from build123d import *

# Parameters (mm, degrees)
SKETCH1_W                 = 610
SKETCH1_H                 = 410
SKETCH1_W_2               = 580
SKETCH1_H_2               = 380
BOSS_EXTRUDE1_DEPTH       = 25
BOSS_EXTRUDE2_DEPTH       = 15
BOSS_EXTRUDE6_DEPTH       = 15
BOSS_EXTRUDE11_DEPTH      = 25
SKETCH8_W                 = 15
SKETCH8_H                 = 130
BOSS_EXTRUDE12_DEPTH      = 25
SKETCH9_W                 = 15
SKETCH9_H                 = 130
BOSS_EXTRUDE13_DEPTH      = 25
SKETCH10_W                = 150
SKETCH10_H                = 25
BOSS_EXTRUDE14_DEPTH      = 15
SKETCH13_W                = 215
SKETCH13_H                = 25
BOSS_EXTRUDE15_DEPTH      = 15
SKETCH14_W                = 215
SKETCH14_H                = 25
BOSS_EXTRUDE16_DEPTH      = 15
BOSS_EXTRUDE17_DEPTH      = 25
BOSS_EXTRUDE17_DEPTH_BACK = 25
BOSS_EXTRUDE17_START      = -205
SKETCH17_W                = 15
SKETCH17_H                = 150
BOSS_EXTRUDE18_DEPTH      = 25
LOFT13_START              = -525.0000001
LOFT13_DEPTH              = 225.0000002
LOFT13_START_2            = -152.5000001
LOFT13_2_DEPTH            = 415.5000001


with BuildPart() as part:
    # Sketch1 → Boss-Extrude1 (new body)
    with BuildSketch(Plane(origin=(0, 0, 0), x_dir=(1, 0, 0), z_dir=(0, 1, 0))):
        with Locations((695.4, -52.5)):
            Rectangle(SKETCH1_W, SKETCH1_H)
        with Locations((695.4, -52.5)):
            Rectangle(SKETCH1_W_2, SKETCH1_H_2, mode=Mode.SUBTRACT)
    extrude(amount=-BOSS_EXTRUDE1_DEPTH)

    # Sketch2 → Boss-Extrude2 (add)
    with BuildSketch(Plane.XY.offset(257.5)):
        Polygon((1000.4, 0), (1000.4, -290), (1190.4, -290), (1190.4, -500), (1165.4, -500), (1165.4, -315), (1000.4, -315), (1000.4, -500), (975.4, -500), (975.4, 0), align=None)
    extrude(amount=-BOSS_EXTRUDE2_DEPTH)

    # Sketch4 → Boss-Extrude6 (add)
    with BuildSketch(Plane(origin=(0, 0, -152.5), x_dir=(-1, 0, 0), z_dir=(0, 0, -1))):
        Polygon((-1000.4, -500), (-1000.4, -315), (-1165.4, -315), (-1165.4, -500), (-1190.4, -500), (-1190.4, -290), (-1000.4, -290), (-1000.4, 0), (-975.4, 0), (-975.4, -500), align=None)
    extrude(amount=-BOSS_EXTRUDE6_DEPTH)

    # Sketch6 → Boss-Extrude11 (add)
    with BuildSketch(Plane(origin=(0, -290, 0), x_dir=(1, 0, 0), z_dir=(0, 1, 0))):
        Polygon((1700.4, 22.5), (1715.4, 22.5), (1715.4, -52.5), (1715.4, -127.5), (1700.4, -127.5), (1190.4, -257.5), (1190.4, -242.5), (1700.4, -112.5), (1700.4, 7.5), (1190.4, 137.5), (1190.4, 152.5), align=None)
    extrude(amount=-BOSS_EXTRUDE11_DEPTH)

    # Sketch8 → Boss-Extrude12 (add)
    with BuildSketch(Plane.XY.offset(127.5)):
        with Locations((1707.9, -355)):
            Rectangle(SKETCH8_W, SKETCH8_H)
    extrude(amount=-BOSS_EXTRUDE12_DEPTH)

    # Sketch9 → Boss-Extrude13 (add)
    with BuildSketch(Plane(origin=(0, 0, -22.5), x_dir=(-1, 0, 0), z_dir=(0, 0, -1))):
        with Locations((-1707.9, -355)):
            Rectangle(SKETCH9_W, SKETCH9_H)
    extrude(amount=-BOSS_EXTRUDE13_DEPTH)

    # Sketch10 → Boss-Extrude14 (add)
    with BuildSketch(Plane.ZY.offset(-1700.4)):
        with Locations((52.5, -407.5)):
            Rectangle(SKETCH10_W, SKETCH10_H)
    extrude(amount=-BOSS_EXTRUDE14_DEPTH)

    # Sketch13 → Boss-Extrude15 (add)
    with BuildSketch(Plane(origin=(0, 0, -152.5), x_dir=(-1, 0, 0), z_dir=(0, 0, -1))):
        with Locations((-1082.9, -512.5)):
            Rectangle(SKETCH13_W, SKETCH13_H)
    extrude(amount=-BOSS_EXTRUDE15_DEPTH)

    # Sketch14 → Boss-Extrude16 (add)
    with BuildSketch(Plane.XY.offset(257.5)):
        with Locations((1082.9, -512.5)):
            Rectangle(SKETCH14_W, SKETCH14_H)
    extrude(amount=-BOSS_EXTRUDE16_DEPTH)

    # Sketch12 → Loft2 section 0
    with BuildSketch(Plane(origin=(1715.4, 0, 0), x_dir=(0, 0, -1), z_dir=(1, 0, 0))):
        with BuildLine():
            Line((22.5, -420), (22.5, -395))
            Line((22.5, -395), (7.5, -395))
            Line((7.5, -395), (7.5, -420))
            Line((7.5, -420), (22.5, -420))
        make_face()
    # Sketch15 → Loft2 section 1
    with BuildSketch(Plane(origin=(1190.4, 0, 0), x_dir=(0, 0, -1), z_dir=(1, 0, 0))):
        with BuildLine():
            Line((152.5, -525), (137.5, -525))
            Line((137.5, -525), (137.5, -500))
            Line((137.5, -500), (152.5, -500))
            Line((152.5, -500), (152.5, -525))
        make_face()
    loft()

    # Sketch18 → Loft3 section 0
    with BuildSketch(Plane(origin=(1715.4, 0, 0), x_dir=(0, 0, -1), z_dir=(1, 0, 0))):
        with BuildLine():
            Line((-127.5, -420), (-112.5, -420))
            Line((-112.5, -420), (-112.5, -395))
            Line((-112.5, -395), (-127.5, -395))
            Line((-127.5, -395), (-127.5, -420))
        make_face()
    # Sketch19 → Loft3 section 1
    with BuildSketch(Plane(origin=(1190.4, 0, 0), x_dir=(0, 0, -1), z_dir=(1, 0, 0))):
        with BuildLine():
            Line((-257.5, -525), (-242.5, -525))
            Line((-242.5, -525), (-242.5, -500))
            Line((-242.5, -500), (-257.5, -500))
            Line((-257.5, -500), (-257.5, -525))
        make_face()
    loft()



with BuildPart() as body_2:
    # Sketch17 → Boss-Extrude17 (new, two sides: drawn at the far end of the back side and taken through both)
    with BuildSketch(Plane.XY.offset(257.5).offset(BOSS_EXTRUDE17_START - BOSS_EXTRUDE17_DEPTH_BACK)):
        with Locations((-912.1, -250)):
            Rectangle(SKETCH17_W, SKETCH17_H)
    extrude(amount=BOSS_EXTRUDE17_DEPTH + BOSS_EXTRUDE17_DEPTH_BACK)


with BuildPart() as part_1:
    add(part.part)

    add(body_2.part)  # Loft6 merges body 2
    # Sketch21 → Loft6 section 0
    with BuildSketch(Plane(origin=(-904.6, 0, 0), x_dir=(0, 0, -1), z_dir=(1, 0, 0))):
        with BuildLine():
            Line((-77.5, -175), (-62.5, -175))
            Line((-62.5, -175), (-62.5, -200))
            Line((-62.5, -200), (-77.5, -200))
            Line((-77.5, -200), (-77.5, -175))
        make_face()
    # Sketch20 → Loft6 section 1
    with BuildSketch(Plane.ZY.offset(-390.4)):
        with BuildLine():
            Line((257.5, 0), (257.5, -25))
            Line((257.5, -25), (242.5, -25))
            Line((242.5, -25), (242.5, 0))
            Line((242.5, 0), (257.5, 0))
        make_face()
    loft()

    # Sketch23 → Loft7 section 0
    with BuildSketch(Plane.ZY.offset(-390.4)):
        with BuildLine():
            Line((-152.5, 0), (-137.5, 0))
            Line((-137.5, 0), (-137.5, -25))
            Line((-137.5, -25), (-152.5, -25))
            Line((-152.5, -25), (-152.5, 0))
        make_face()
    # Sketch22 → Loft7 section 1
    with BuildSketch(Plane(origin=(-904.6, 0, 0), x_dir=(0, 0, -1), z_dir=(1, 0, 0))):
        with BuildLine():
            Line((-27.5, -175), (-27.5, -200))
            Line((-27.5, -200), (-42.5, -200))
            Line((-42.5, -200), (-42.5, -175))
            Line((-42.5, -175), (-27.5, -175))
        make_face()
    loft()

    # Sketch24 → Boss-Extrude18 (add)
    with BuildSketch(Plane.XZ.offset(525)):
        Polygon((975.4, 257.5), (765.4, 257.5), (765.4, -152.5), (975.4, -152.5), (975.4, -137.5), (780.4, -137.5), (780.4, 242.5), (975.4, 242.5), align=None)
    extrude(amount=-BOSS_EXTRUDE18_DEPTH)

    # Loft13: read off the stored shape, not the designer's step
    # Loft13 outline → Loft13 (add)
    with BuildSketch(Plane(origin=(0, 0, 0), x_dir=(1, 0, 0), z_dir=(0, 1, 0)).offset(LOFT13_START)):
        with BuildLine():
            Line((-904.6, -62.5), (-904.6, -77.5))
            add(Edge.make_bspline(
                [(-904.6, -77.5), (-764.041130949, -75.679060612), (-527.584659858, -129.428121998), (-157.569765668, -171.662088503), (257.177772802, -240.107254931), (577.127812515, -271.097379608), (765.4, -257.5)],
                knots=[0, 0, 0, 0, 0.250527251, 0.428009069, 0.664938737, 1, 1, 1, 1], degree=3))
            Line((765.4, -257.5), (765.4, -242.5))
            add(Edge.make_bspline(
                [(-904.6, -62.5), (-764.041130949, -60.679060612), (-527.584659858, -114.428121998), (-157.569765668, -156.662088503), (257.177772802, -225.107254931), (577.127812515, -256.097379608), (765.4, -242.5)],
                knots=[0, 0, 0, 0, 0.250527251, 0.428009069, 0.664938737, 1, 1, 1, 1], degree=3))
        make_face()
    extrude(amount=LOFT13_DEPTH)

    # Loft13 2 outline → Loft13 2 (cut)
    with BuildSketch(Plane.XY.offset(LOFT13_START_2)):
        Polygon((-904.6, -300), (765.4, -500), (765.4, -299.9999999), align=None)
        Polygon((765.4, -525), (-904.6, -325), (-904.6, -525.0000001), align=None)
    extrude(amount=LOFT13_2_DEPTH, mode=Mode.SUBTRACT)


solid = part_1.part
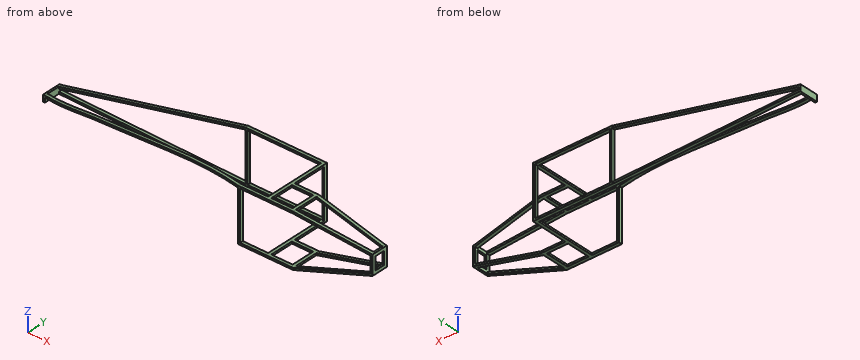
Could you check a few things on this model? Use its own coordinates, in mm. Give positions to 0.01 mm unless a question says otherwise; leave off trailing zeros. Write each loop counter-clockwise with the first axis right and the second up, starting at its lowest first coordinate (ties: lowest second). Pieces come first, ordered by that corner, then holes. Notation, with made-up numbers: (-25, 86.25) -> (-1, 86.25) arc R23 ccw to (-1, 118.25) -> close; hole circle Ø4 at (18, 25.5). An arc over 180 degrees is marked (long way). Answer as a JSON object with one key per item and string values.
Q1. Please list where these lines run through material, in increasing order: L1, parallel to X at y = -409, z = -1; L2, parallel to X at y = -206, z = 47; L3, parallel to Y at x = 285, z = -128.5.
Taken from the geometry:
{"L1": "x = 1700.4 to 1715.4", "L2": "x = -919.6 to -904.6", "L3": "y = -39.24 to -14.24"}
Q2. Will these pins go through, and if not, where does the flat tip stop? pin 1 Ø15 at (y, z) = (-257.5, 44) entering from +X; pin 2 Ø16.5 at (x, z) = (1120.5, 250) entering from +Y; pin 3 Ø4.5 at (y, z) = (-182, 248.5) entering from -X.
Taken from the geometry:
{"pin 1": "stops at x = -904.6", "pin 2": "stops at y = -290", "pin 3": "stops at x = 975.4"}
Q3. Suppose I cut it at B-B on x = 868. Write out the boundary of the cut face in (y, z), then the cut area to 3 significant figures.
Taken from the geometry:
{"outline": "(-525, -152.5) -> (-500, -152.5) -> (-500, -137.5) -> (-525, -137.5) -> close; (-525, 242.5) -> (-500, 242.5) -> (-500, 257.5) -> (-525, 257.5) -> close; (-25, -152.5) -> (0, -152.5) -> (0, -137.5) -> (-25, -137.5) -> close; (-25, 242.5) -> (0, 242.5) -> (0, 257.5) -> (-25, 257.5) -> close", "area": "1,500 mm²"}
Q4. Suppose I cut it at A-A on y = -237. Write out the boundary of the cut face in (x, z), then the cut area to 3 significant figures.
Taken from the geometry:
{"outline": "(-919.6, 27.5) -> (-904.6, 27.5) -> (-904.6, 77.5) -> (-919.6, 77.5) -> close; (975.4, -152.5) -> (1000.4, -152.5) -> (1000.4, -137.5) -> (975.4, -137.5) -> close; (975.4, 242.5) -> (1000.4, 242.5) -> (1000.4, 257.5) -> (975.4, 257.5) -> close", "area": "1,500 mm²"}
